```python
from build123d import *

# Parameters (mm, degrees)
SKETCH1_R               = 4
BOSS_EXTRUDE1_DEPTH     = 24.5
FILLET1_R               = 4
M6_CLEARANCE_HOLE1_D    = 6.6
M2_CLEARANCE_HOLE1_D    = 2.4
CUT_EXTRUDE1_DEPTH      = 40.172694572
CUT_EXTRUDE1_DEPTH_BACK = 40.172694572
FILLET3_R               = 3
FILLET4_R               = 1


with BuildPart() as part:
    # Sketch1 → Boss-Extrude1 (new, symmetric)
    with BuildSketch(Plane.XY):
        with Locations((-25.5, 0)):
            Circle(SKETCH1_R)
        with BuildLine():
            Line((0, 4), (-25.5, 4))
            ThreePointArc((-25.5, 4), (-22.671572875, 2.828427125), (-21.5, 0))
            Line((-21.5, 0), (0, 0))
            Line((0, 0), (0, 4))
        make_face()
        with BuildLine():
            Line((25.5, 4), (0, 4))
            Line((0, 4), (0, 0))
            Line((0, 0), (21.5, 0))
            ThreePointArc((21.5, 0), (22.671572875, 2.828427125), (25.5, 4))
        make_face()
        with Locations((25.5, 0)):
            Circle(SKETCH1_R)
    extrude(amount=BOSS_EXTRUDE1_DEPTH, both=True)

    # Fillet1
    fillet1_edges = [part.edges().sort_by_distance(p)[0] for p in [
        (21.5, 0, 0),
        (-21.5, 0, 0),
    ]]
    fillet(fillet1_edges, radius=FILLET1_R)

    # M6 Clearance Hole1 (through all)
    with Locations(Plane.XY.offset(24.5)):
        with Locations((-25.5, 0), (25.5, 0)):
            Hole(M6_CLEARANCE_HOLE1_D / 2)

    # M2 Clearance Hole1 (through all)
    with Locations(Plane(origin=(0, 4, 0), x_dir=(1, 0, 0), z_dir=(0, 1, 0))):
        with Locations((-7, 10.5), (7, 10.5), (7, -10.5), (-7, -10.5)):
            Hole(M2_CLEARANCE_HOLE1_D / 2)

    # Sketch6 → Cut-Extrude1 (cut, two sides: drawn at the far end of the back side and taken through both)
    with BuildSketch(Plane(origin=(0, 4, 0), x_dir=(1, 0, 0), z_dir=(0, 1, 0)).offset(-CUT_EXTRUDE1_DEPTH_BACK)):
        Polygon((18.57179677, 24.5), (0, 24.5), (0, 14.5), (8.57179677, 14.5), align=None)
        Polygon((0, 24.5), (-18.57179677, 24.5), (-8.57179677, 14.5), (0, 14.5), align=None)
        Polygon((18.57179677, -17.428932188), (11.07179677, -9.928932188), (11.07179677, 9.928932188), (18.57179677, 17.428932188), align=None)
        Polygon((-8.57179677, -14.5), (-18.57179677, -24.5), (18.57179677, -24.5), (8.57179677, -14.5), align=None)
        Polygon((-16.07179677, 14.928932188), (-18.57179677, 17.428932188), (-18.57179677, 0.003413414), (-18.57179677, -0.003413414), (-18.57179677, -17.428932188), (-16.07179677, -14.928932188), align=None)
    extrude(amount=CUT_EXTRUDE1_DEPTH + CUT_EXTRUDE1_DEPTH_BACK, mode=Mode.SUBTRACT)

    # Fillet3
    fillet3_edges = [part.edges().sort_by_distance(p)[0] for p in [
        (18.57179677, 2, -17.428932188),
        (18.57179677, 2, 17.428932188),
        (11.07179677, 2, 9.928932188),
        (11.07179677, 2, -9.928932188),
        (18.57179677, 2, -24.5),
        (8.57179677, 2, -14.5),
        (-8.57179677, 2, -14.5),
        (-18.57179677, 2, -24.5),
        (-8.57179677, 2, 14.5),
        (8.57179677, 2, 14.5),
        (18.57179677, 2, 24.5),
        (-18.57179677, 2, 24.5),
    ]]
    fillet(fillet3_edges, radius=FILLET3_R)

    # Fillet4
    fillet4_edges = [part.edges().sort_by_distance(p)[0] for p in [
        (-18.57179677, 2, 17.428932188),
        (-18.57179677, 2, -17.428932188),
        (-16.07179677, 2, -14.928932188),
        (-16.07179677, 2, 14.928932188),
    ]]
    fillet(fillet4_edges, radius=FILLET4_R)


solid = part.part
```
Geometry: final body of the model. Coordinates: model frame, mm. A direction names the side the tool comes from. Round coordinates to 2 decimals unless told otherwise and drop trailing zeros. Write each loop counter-clockwise with the first axis right and the second up, starting at its lowest first coordinate (ties: lowest second). Pieces come first, ordered by that corner, then holes. Notation, with made-up numbers: M 36,59 L 81,59 A17 ccw 81,83 Z; hole C 43.25,-20 d7. An arc over 180 degrees is marked long. Answer in a Markdown table with one row per item. Add a question column.
(1) Cut plane A-A, the plane z = -19.5. Return the cut outline in (x, y), then the cut area to 3 significant figures.
(2) Cut plane B-B, the plane z = 3. Return the cut outline in (x, y), then the cut area to 3 significant figures.
(3) Ray query, L1, parallel to Z at x = -7, y = 1.15; L2, parallel to Y at x = -25.5, z = 13.5; L3, parallel to X at y = 2.75, z = -2.5. Return the intervals inside material, ascending.
(4) Reachability of faces 1 (the face through (-16.072, 2, 0)), 2 (the face through (13.63, 1.97, 19.56)), 3 (the face through (18.651, 1.93, -24.265)) from +Z, -Z, +X, -X, +Y, -Y: full face, straight path, thin tool, end or side. Return the list, or none.
(5) Contact query for flat-ended pins moving along their axis: pin 1 (1.2 mm diameter, centred on y = 3, z = -1, fed in from +X); pin 2 (3 mm diameter, centred on y = 1.5, z = -3, fed in from +X); pin 3 (1.9 mm diameter, centred on x = 7, z = 10.5, fed in from +Y); pin 4 (1.5 mm diameter, centred on x = 18, z = -16, fed in from -Y). Output: stop coordinate, or through.
(6) Draft query along X for faces 4 (the face through (-17.97, 2.03, 15.93)), 5 (the face through (-22.57, 1.83, -24.5)). Return one class per face: pulls with the +X half, pulls with the -X half, needs draft (parallel to the pull), parting line crosses it, or undercut.
(7) Cut plane D-D, the plane x = -1. Return the cut outline in (y, z), then the cut area to 3 significant figures.
(8) Cut plane C-C, the plane y = -1. Return the cut outline in (x, z).
Established:
| question | item | result |
|---|---|---|
| 1 | outline | M -25.5,4 A4 ccw long -22.04,-2 A4 cw -18.57,0 L -13.57,0 L -13.57,4 Z; M 13.57,0 L 18.57,0 A4 cw 22.04,-2 A4 ccw long 25.5,4 L 13.57,4 Z; hole C -25.5,0 d6.6; hole C 25.5,0 d6.6 |
| 1 | area | 105 mm² |
| 2 | outline | M -25.5,4 A4 ccw long -22.04,-2 A4 cw -18.57,0 L -18.57,4 Z; M -16.07,0 L 11.07,0 L 11.07,4 L -16.07,4 Z; M 18.57,0 A4 cw 22.04,-2 A4 ccw long 25.5,4 L 18.57,4 Z; hole C -25.5,0 d6.6; hole C 25.5,0 d6.6 |
| 2 | area | 174 mm² |
| 3 | L1 | -14.5 to -11.7, -9.3 to 9.3, 11.7 to 14.5 |
| 3 | L2 | -4 to -3.3, 3.3 to 4 |
| 3 | L3 | -28.4 to -27.32, -23.68 to -18.57, -16.07 to 11.07, 18.57 to 23.68, 27.32 to 28.4 |
| 4 | face 1 | +Y, -Y |
| 4 | face 2 | +Z, +Y, -Y |
| 4 | face 3 | -Z, +Y, -Y |
| 5 | pin 1 | x = 28.7 |
| 5 | pin 2 | x = 29.5 |
| 5 | pin 3 | through |
| 5 | pin 4 | y = 0 |
| 6 | face 4 | undercut |
| 6 | face 5 | needs draft |
| 7 | outline | M 0,-14.5 L 4,-14.5 L 4,14.5 L 0,14.5 Z |
| 7 | area | 116 mm² |
| 8 | outline | M -29.37,-24.5 L -28.64,-24.5 L -28.64,24.5 L -29.37,24.5 Z; M -22.36,-24.5 L -21.22,-24.5 L -21.22,24.5 L -22.36,24.5 Z; M 21.22,-24.5 L 22.36,-24.5 L 22.36,24.5 L 21.22,24.5 Z; M 28.64,-24.5 L 29.37,-24.5 L 29.37,24.5 L 28.64,24.5 Z |
